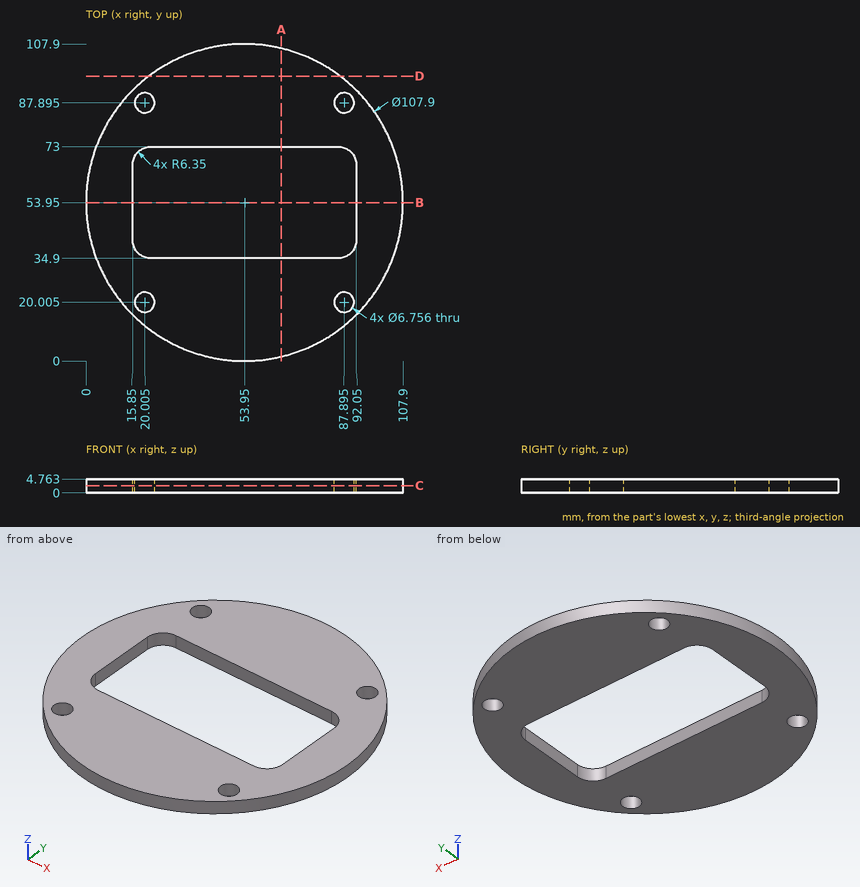
The drawing under review shows one solid part. Ordinate dimensions are in mm from its lowest x, y, z. Give positions to 0.01 mm unless a question says otherwise; leave off trailing zeros. Order: outer loops, then holes, each group sorted by start corner. A loop starts at its lowest first (then second) coordinate and runs counter-clockwise, first axis right, second up. Notation, with made-up numbers: (72, 38) -> (120, 38) arc R31 cw to (120, 76) -> close; hole circle Ø1 at (-1.5, 48.5). An arc over 180 degrees is marked (long way). Write item = value, one per line. Start each with the question number.
(1) We need section C-C on z = 2.55. State how many separate pieces and enclosed holes the cut face has, plus the area to 3 significant figures.
(2) We need section D-D on y = 97. Write out the cut boundary in (x, z).
(3) To check wall thickness, follow line 1 along Y through (x, z) = (89, 0.9) (1 decimal); line 2 along Y through (x, z) = (53, 1.3); line 3 along Y through (x, z) = (36.5, 1.3). State the ranges of each line that lie inside material, in increasing order.
(4) We need section B-B on y = 53.95. Write out the cut boundary in (x, z).
(5) For pin 1 (1.5 mm diameter, centred on x = 14.5, y = 34.5, fed in from -Z); pin 2 (2.5 mm diameter, centred on x = 53.5, z = 1.5, fed in from -Y); pin 3 (1.4 mm diameter, centred on y = 51, z = 3.5, fed in from -X); pin 4 (2.5 mm diameter, centred on y = 57, z = 2.5, fed in from +X), all flat-tipped, find the tip position at first contact; note any pin that passes through.
(6) We need section A-A on x = 66.5. Write out the cut boundary in (y, z).
Numbers:
q1.separate_pieces = 1
q1.enclosed_holes = 5
q1.area = 6,130 mm^2
q2.outline = (21.43, 0) -> (86.47, 0) -> (86.47, 4.76) -> (21.43, 4.76) -> close
q3.line_1 = 12.9 to 16.8, 23.2 to 35.8, 72.1 to 84.7, 91.1 to 95
q3.line_2 = 0.01 to 34.9, 73 to 107.89
q3.line_3 = 2.9 to 34.9, 73 to 105
q4.outline = (0, 0) -> (15.85, 0) -> (15.85, 4.76) -> (0, 4.76) -> close; (92.05, 0) -> (107.9, 0) -> (107.9, 4.76) -> (92.05, 4.76) -> close
q5.pin_1 = 0
q5.pin_2 = 0
q5.pin_3 = 0.05
q5.pin_4 = 107.87
q6.outline = (1.48, 0) -> (34.9, 0) -> (34.9, 4.76) -> (1.48, 4.76) -> close; (73, 0) -> (106.42, 0) -> (106.42, 4.76) -> (73, 4.76) -> close
